```python
from build123d import *

# Parameters (mm, degrees)
F0_W             = 20
F0_H             = 20
F1_DEPTH         = 520
F2_R             = 2.1
F3_DEPTH         = 520.001
F4_R             = 1
F6_DEPTH         = 520.001
F6_COPIES3_COUNT = 2
F6_COPIES3_ANGLE = 90
F6_COPIES4_COUNT = 2
F6_COPIES4_ANGLE = 270
F6_COPIES6_COUNT = 2
F9_W             = 16.4
F9_H             = 6.8613203436
F10_DEPTH        = 520.001
F12_DEPTH        = 520


# Not quite as in the source:
# - a pattern or mirror of a feature is missing from the dataset's text; its kind, count and spacing are read off the source's solid


with BuildPart() as f1:
    # F0 (on Front) → F1 (new body)
    with BuildSketch(Plane.XZ):
        Rectangle(F0_W, F0_H)
    extrude(amount=F1_DEPTH)

    # F2 (on face) → F3 (cut, through all)
    with BuildSketch(Plane.XZ.offset(520)):
        Circle(F2_R)
    extrude(amount=-F3_DEPTH, mode=Mode.SUBTRACT)

    # F4
    f4_edges = [f1.edges().sort_by_distance(p)[0] for p in [
        (-10, -260, 10),
        (10, -260, 10),
    ]]
    fillet(f4_edges, radius=F4_R)

    # F5 (on face) → F6 (cut, through all)
    with BuildSketch(Plane.XZ.offset(520)):
        Polygon((0, 3.9006601718), (0, 10), (-2.84, 10), (-4.64, 10), (-2.84, 8.2), (-5.4993398282, 8.2), (-5.4993398282, 6.56), (-2.84, 3.9006601718), align=None)
        Polygon((-6.5693398282, 8.2), (-8.2, 8.2), (-7.0953059148, 7.0953059148), (-6.5693398282, 7.6212720014), align=None)
    f6 = extrude(amount=-F6_DEPTH, mode=Mode.SUBTRACT)

    # F6_copies: F6 across plane
    add(f6.mirror(Plane(origin=(0, 0, 0), x_dir=(-0.7071067812, 0, -0.7071067812), z_dir=(0.7071067812, 0, -0.7071067812))), mode=Mode.SUBTRACT)

    # F6_copies1: F6 across plane
    add(f6.mirror(Plane(origin=(0, 0, 0), x_dir=(0.7071067812, 0, -0.7071067812), z_dir=(-0.7071067812, 0, -0.7071067812))), mode=Mode.SUBTRACT)

    # F6_copies2: F6 across plane
    add(f6.mirror(Plane(origin=(0, 0, 0), x_dir=(0, 0, 1), z_dir=(1, 0, 0))), mode=Mode.SUBTRACT)

    # F6_copies3: F6 ×2 about axis
    f6_copies3_axis = Axis((0, 0, 0), (0, 1, 0))
    for i in range(1, F6_COPIES3_COUNT):
        add(f6.rotate(f6_copies3_axis, i * F6_COPIES3_ANGLE / (F6_COPIES3_COUNT - 1)), mode=Mode.SUBTRACT)

    # F6_copies4: F6 ×2 about axis
    f6_copies4_axis = Axis((0, 0, 0), (0, 1, 0))
    for i in range(1, F6_COPIES4_COUNT):
        add(f6.rotate(f6_copies4_axis, i * F6_COPIES4_ANGLE / (F6_COPIES4_COUNT - 1)), mode=Mode.SUBTRACT)

    # F6_copies5: F6 across plane
    add(f6.mirror(Plane(origin=(0, 0, 0), x_dir=(-1, 0, 0), z_dir=(0, 0, -1))), mode=Mode.SUBTRACT)

    # F6_copies6: F6 ×2 about axis
    f6_copies6_axis = Axis((0, 0, 0), (0, 1, 0))
    for i in range(1, F6_COPIES6_COUNT):
        add(f6.rotate(f6_copies6_axis, i * 360 / F6_COPIES6_COUNT), mode=Mode.SUBTRACT)

    # F8: F1 across face


with BuildPart() as f1_1:
    add(f1.part)
    add(f1.part.mirror(Plane(origin=(-7.32, -260, -10), x_dir=(1, 0, 0), z_dir=(0, 0, -1))))

    # F9 (on face) → F10 (cut, through all)
    with BuildSketch(Plane.XZ.offset(520)):
        with Locations((0, -10)):
            Rectangle(F9_W, F9_H)
    extrude(amount=-F10_DEPTH, mode=Mode.SUBTRACT)

    # F11 (on face) → F12 (join, through all)
    with BuildSketch(Plane.XZ.offset(520)):
        with BuildLine():
            ThreePointArc((-9, -10), (-9.7071067812, -9.7071067812), (-10, -9))
            Line((-10, -9), (-10, -11))
            ThreePointArc((-10, -11), (-9.7071067812, -10.2928932188), (-9, -10))
        make_face()
        with BuildLine():
            ThreePointArc((10, -9), (9.7071067812, -9.7071067812), (9, -10))
            ThreePointArc((9, -10), (9.7071067812, -10.2928932188), (10, -11))
            Line((10, -11), (10, -9))
        make_face()
        Polygon((5.9386796564, -6.9993398282), (8.2, -6.9993398282), (8.2, -6.5693398282), (5.5086796564, -6.5693398282), align=None)
        Polygon((-8.2, -6.5693398282), (-8.2, -6.9993398282), (-5.9386796564, -6.9993398282), (-5.5086796564, -6.5693398282), align=None)
    extrude(amount=-F12_DEPTH)


solid = f1_1.part
```
Read the model definition and answer for the solid it produces. Units are mm, in the model's axes. Coordinates: 2 decimals unless noted, no trailing zeros. Answer as a JSON object with one key per item and string values.
Q1. Flat-ended cylindrical pins translate along their axes: pin 1 Ø6 at (x, y) = (-1, -376.5) entering from +Z; pin 2 Ø3 at (y, z) = (-180.5, -1) entering from +X; pin 3 Ø6 at (y, z) = (-435, -20.5) entering from +X. Find the tip coordinate at first contact, or state that the pin passes through.
The answers:
{"pin 1": "stops at z = 9.36", "pin 2": "stops at x = 3.9", "pin 3": "stops at x = 8.86"}
Q2. The part is cut by section A-A on y = -133.5. Give the number of separate pieces and of enclosed holes in the cut face, then the cut area to 3 significant figures.
The answers:
{"separate pieces": "1", "enclosed holes": "7", "area": "286 mm2"}
Q3. Consider line 1 (Z direction, x = 0, y = -351.5); line 2 (X direction, y = -255, z = -20); line 3 (Z direction, x = 5.75, y = -189). Determine where each line is inside the solid, lowest interval first. Write a range as [from, to].
The answers:
{"line 1": "z = [-23.9, -22.1], [-17.9, -16.1], [-3.9, -2.1], [2.1, 3.9]", "line 2": "x = [-3.9, -2.1], [2.1, 3.9]", "line 3": "z = [-30, -24.69], [-15.31, -13.43], [-6.81, -4.69], [4.69, 10]"}
